Geometry: final body of the model. Coordinates: model frame, mm. A direction names the side the tool comes from. Coordinates: 2 decimals unless noted, no trailing zeros. Write each loop counter-clockwise with the first axis right and the second up, starting at its lowest first coordinate (ties: lowest second). Pieces come first, ordered by that corner, then holes. Notation, with made-up numbers: (-25.5, 10.5) - (-0.5, 10.5) arc R10 cw to (-0.5, 20.5) - close; hole circle Ø9 at (17, 2). An arc over 180 degrees is marked (long way). Answer as a JSON object with one key per item and string values. Group by question number.
Item 1: Set-up query: faces 3 (the flat face through (103, 106, 3)), 4 (the flat face through (148.76, 54.52, 1.48)). Return all of +Z, -Z, +X, -X, +Y, -Y with unobstructed straight access to the full face (end or side cutting, diameter ignored); none if empty.
Item 2: Section A-A on y = 121. Return loops of the section in (x, z), and give its area (3 significant figures).
Item 3: Mould query, pull axis X, two halves, no side actions, for faces 1 (the flat face through (103, 106, 0)), 2 (the flat face through (55.659, 44.946, 1.479)). Classes: pulls with the +X half, pulls with the -X half, needs draft (parallel to the pull), parting line crosses it, or undercut.
Item 4: Section B-B on x = 141.5. Return loops of the section in (y, z), and give its area (3 significant figures).
Item 5: Section C-C on y = 179. Return loops of the section in (x, z), and give its area (3 significant figures).
Item 6: Section D-D on z = 2.45. State how many separate pieces and enclosed holes the cut face has, and give its area (3 significant figures).
Item 7: Line query: line 1 along X through (y, z) = (113, 0.7); line 2 along Y through (x, z) = (2.5, 1.55); line 3 along Y through (x, z) = (113, 1.15). Output: solid intervals per line, ascending. Write a range as from..to.
```python
from build123d import *

# Parameters (mm, degrees)
SKETCH_1_R      = 1.6
EXTRUDE_1_DEPTH = 3


with BuildPart() as part:
    # 草图1 → 凸台-拉伸1 (new body)
    with BuildSketch(Plane.XY):
        with BuildLine():
            Line((2, 0), (207, 0))
            ThreePointArc((207, 0), (208.414213562, 0.585786438), (209, 2))
            Line((209, 2), (209, 208))
            ThreePointArc((209, 208), (208.414213562, 209.414213562), (207, 210))
            Line((207, 210), (2, 210))
            ThreePointArc((2, 210), (0.585786438, 209.414213562), (0, 208))
            Line((0, 208), (0, 2))
            ThreePointArc((0, 2), (0.585786438, 0.585786438), (2, 0))
        make_face()
        with Locations((2.5, 97)):
            Circle(SKETCH_1_R, mode=Mode.SUBTRACT)
        with Locations((17.5, 97)):
            Circle(SKETCH_1_R, mode=Mode.SUBTRACT)
        with Locations(Location((17.5, 113, 0), (0, 0, 180))):
            Circle(SKETCH_1_R, mode=Mode.SUBTRACT)
        with Locations(Location((2.5, 113, 0), (0, 0, 180))):
            Circle(SKETCH_1_R, mode=Mode.SUBTRACT)
        with Locations(Location((206.5, 97, 0), (0, 0, 180))):
            Circle(SKETCH_1_R, mode=Mode.SUBTRACT)
        with Locations(Location((191.5, 97, 0), (0, 0, 180))):
            Circle(SKETCH_1_R, mode=Mode.SUBTRACT)
        with Locations((191.5, 113)):
            Circle(SKETCH_1_R, mode=Mode.SUBTRACT)
        with Locations((206.5, 113)):
            Circle(SKETCH_1_R, mode=Mode.SUBTRACT)
        with BuildLine():
            Line((24.808355785, 95), (97.5, 95))
            ThreePointArc((97.5, 95), (98.914213562, 94.414213562), (99.5, 93))
            Line((99.5, 93), (99.5, 19.878227713))
            ThreePointArc((99.5, 19.878227713), (98.262640733, 18.029341802), (96.081620887, 18.468192007))
            Line((96.081620887, 18.468192007), (23.389976673, 91.589964294))
            ThreePointArc((23.389976673, 91.589964294), (22.961727586, 93.768091332), (24.808355785, 95))
        make_face(mode=Mode.SUBTRACT)
        with BuildLine():
            Line((112.918379113, 18.468192007), (185.610023327, 91.589964294))
            ThreePointArc((185.610023327, 91.589964294), (186.038272414, 93.768091332), (184.191644215, 95))
            Line((184.191644215, 95), (111.5, 95))
            ThreePointArc((111.5, 95), (110.085786438, 94.414213562), (109.5, 93))
            Line((109.5, 93), (109.5, 19.878227713))
            ThreePointArc((109.5, 19.878227713), (110.737359267, 18.029341802), (112.918379113, 18.468192007))
        make_face(mode=Mode.SUBTRACT)
        with BuildLine():
            Line((20, 75.967320112), (20, 12))
            ThreePointArc((20, 12), (20.585786438, 10.585786438), (22, 10))
            Line((22, 10), (85.591041759, 10))
            ThreePointArc((85.591041759, 10), (87.437669958, 11.231908668), (87.009420872, 13.410035706))
            Line((87.009420872, 13.410035706), (23.418379113, 77.377355819))
            ThreePointArc((23.418379113, 77.377355819), (21.237359267, 77.816206024), (20, 75.967320112))
        make_face(mode=Mode.SUBTRACT)
        with BuildLine():
            Line((121.990579128, 13.410035706), (185.581620887, 77.377355819))
            ThreePointArc((185.581620887, 77.377355819), (187.762640733, 77.816206024), (189, 75.967320112))
            Line((189, 75.967320112), (189, 12))
            ThreePointArc((189, 12), (188.414213562, 10.585786438), (187, 10))
            Line((187, 10), (123.408958241, 10))
            ThreePointArc((123.408958241, 10), (121.562330042, 11.231908668), (121.990579128, 13.410035706))
        make_face(mode=Mode.SUBTRACT)
        with BuildLine():
            Line((187, 200), (123.408958241, 200))
            ThreePointArc((123.408958241, 200), (121.562330042, 198.768091332), (121.990579128, 196.589964294))
            Line((121.990579128, 196.589964294), (185.581620887, 132.622644181))
            ThreePointArc((185.581620887, 132.622644181), (187.762640733, 132.183793976), (189, 134.032679888))
            Line((189, 134.032679888), (189, 198))
            ThreePointArc((189, 198), (188.414213562, 199.414213562), (187, 200))
        make_face(mode=Mode.SUBTRACT)
        with BuildLine():
            Line((87.009420872, 196.589964294), (23.418379113, 132.622644181))
            ThreePointArc((23.418379113, 132.622644181), (21.237359267, 132.183793976), (20, 134.032679888))
            Line((20, 134.032679888), (20, 198))
            ThreePointArc((20, 198), (20.585786438, 199.414213562), (22, 200))
            Line((22, 200), (85.591041759, 200))
            ThreePointArc((85.591041759, 200), (87.437669958, 198.768091332), (87.009420872, 196.589964294))
        make_face(mode=Mode.SUBTRACT)
        with BuildLine():
            Line((184.191644215, 115), (111.5, 115))
            ThreePointArc((111.5, 115), (110.085786438, 115.585786438), (109.5, 117))
            Line((109.5, 117), (109.5, 190.121772287))
            ThreePointArc((109.5, 190.121772287), (110.737359267, 191.970658198), (112.918379113, 191.531807993))
            Line((112.918379113, 191.531807993), (185.610023327, 118.410035706))
            ThreePointArc((185.610023327, 118.410035706), (186.038272414, 116.231908668), (184.191644215, 115))
        make_face(mode=Mode.SUBTRACT)
        with BuildLine():
            Line((23.389976673, 118.410035706), (96.081620887, 191.531807993))
            ThreePointArc((96.081620887, 191.531807993), (98.262640733, 191.970658198), (99.5, 190.121772287))
            Line((99.5, 190.121772287), (99.5, 117))
            ThreePointArc((99.5, 117), (98.914213562, 115.585786438), (97.5, 115))
            Line((97.5, 115), (24.808355785, 115))
            ThreePointArc((24.808355785, 115), (22.961727586, 116.231908668), (23.389976673, 118.410035706))
        make_face(mode=Mode.SUBTRACT)
    extrude(amount=EXTRUDE_1_DEPTH)


solid = part.part
```
Checks:
{
 "1": {"face 3": "+Z, +X, -X, +Y, -Y", "face 4": "+Z, -Z"},
 "2": {"outline": "(0, 0) - (25.96, 0) - (25.96, 3) - (0, 3) - close; (99.5, 0) - (109.5, 0) - (109.5, 3) - (99.5, 3) - close; (183.04, 0) - (209, 0) - (209, 3) - (183.04, 3) - close", "area": "186 mm^2"},
 "3": {"face 1": "needs draft", "face 2": "undercut"},
 "4": {"outline": "(0, 0) - (10, 0) - (10, 3) - (0, 3) - close; (33.03, 0) - (47.22, 0) - (47.22, 3) - (33.03, 3) - close; (95, 0) - (115, 0) - (115, 3) - (95, 3) - close; (162.78, 0) - (176.97, 0) - (176.97, 3) - (162.78, 3) - close; (200, 0) - (210, 0) - (210, 3) - (200, 3) - close", "area": "205 mm^2"},
 "5": {"outline": "(0, 0) - (20, 0) - (20, 3) - (0, 3) - close; (69.52, 0) - (83.62, 0) - (83.62, 3) - (69.52, 3) - close; (99.5, 0) - (109.5, 0) - (109.5, 3) - (99.5, 3) - close; (125.38, 0) - (139.48, 0) - (139.48, 3) - (125.38, 3) - close; (189, 0) - (209, 0) - (209, 3) - (189, 3) - close", "area": "235 mm^2"},
 "6": {"separate pieces": "1", "enclosed holes": "16", "area": "21,200 mm^2"},
 "7": {"line 1": "0..0.9, 4.1..15.9, 19.1..189.9, 193.1..204.9, 208.1..209", "line 2": "0..95.4, 98.6..111.4, 114.6..210", "line 3": "0..18.55, 95..115, 191.45..210"}
}
